Geometry: final body of the model. Coordinates: model frame, mm. A direction names the side the tool comes from. Give positions to 0.01 mm unless a question says otherwise; leave off trailing zeros. Write each loop counter-clockwise with the first axis right and the second up, starting at its lowest first coordinate (ties: lowest second). Pieces come first, ordered by that corner, then holes. Notation, with made-up numbers: (12, 22.5) -> (44, 22.5) arc R13 ccw to (44, 33.5) -> close; hole circle Ø8 at (43, 69.5). An arc over 180 degrees is marked (long way). Answer as a JSON object with one key per item and string values. Group by question number.
(1) Section query D-D on z = 1.75. Output: boundary loops of the cut face in (x, y).
(2) Set-up query: faces 4 (the face through (2, -2, 0)), 5 (the face through (-2, 2, 17)), 6 (the face through (-2.003, 0.631, 2.218)). Return all of +Z, -Z, +X, -X, +Y, -Y with unobstructed straight access to the full face (end or side cutting, diameter ignored); none if empty.
(3) Section query C-C on z = 7.5. Output: boundary loops of the cut face in (x, y), plus the area to 3 significant figures.
(4) Draft query along X for faces 1 (the face through (-3, 0, 20)), 2 (the face through (1, -1, 23)), 3 (the face through (0, -1, 14)). Return one class per face: +X half, -X half, draft (parallel to the pull), parting line (faces both ways), or undercut.
(5) Section query A-A on y = 0. Output: boundary loops of the cut face in (x, z), plus the area to 3 significant figures.
(6) Contact query for flat-ended pins moving along their axis: pin 1 Ø1.6 at (x, y) = (0, 0) entering from -Z; pin 2 Ø2 at (y, z) = (-0.5, 20.5) entering from -X; pin 3 Ø1.3 at (x, y) = (-0.5, 1) entering from -Z; pin 4 Ø1.5 at (x, z) = (1.5, 19) entering from +Y. Output: stop coordinate, or through.
(7) Material intervals for probe 1 along Y at (x, z) = (0, 12); probe 2 along Y at (x, z) = (0, 2.8); probe 3 along Z at (x, y) = (-1.5, 2.75), sorted ascending.
Autodesk Inventor part; units mm, degrees
ref_plane "YZ Plane" through (0, 0, 0) normal (1, 0, 0) x (0, 1, 0)
ref_plane "XZ Plane" through (0, 0, 0) normal (0, 1, 0) x (-1, 0, 0)
ref_plane "XY Plane" through (0, 0, 0) normal (0, 0, 1) x (1, 0, 0)
sketch "Sketch1" plane through (0, 0, 0) normal (0, 0, 1) x (1, 0, 0)
  circle A0 centre (0, 0) radius 3.5
  dimension "d0" = 7
extrude "Extrusion1" add sketch "Sketch1" along normal blind 15
sketch "Sketch2" plane through (0, 0, 15) normal (0, 0, 1) x (1, 0, 0)
  circle A0 centre (0, 0) radius 2.5
  dimension "d3" = 5
extrude "Extrusion2" add sketch "Sketch2" along normal blind 2
sketch "Sketch3" plane through (0, 0, 17) normal (0, 0, 1) x (1, 0, 0)
  circle A0 centre (0, 0) radius 3
  dimension "d6" = 6
extrude "Extrusion3" add sketch "Sketch3" along normal blind 6
sketch "Sketch4" plane through (0, 0, 23) normal (0, 0, 1) x (1, 0, 0)
  circle A0 centre (0, 0) radius 1
  dimension "d9" = 2
extrude "Extrusion4" cut sketch "Sketch4" against normal through all
thread "Thread1"
fillet "Fillet1" radius 0.5 1 edges at (-3, 0, 23)
sketch "Sketch5" plane through (0, 0, 0) normal (0, 0, -1) x (-1, 0, 0)
  circle A0 centre (0, 0) radius 2.1
  dimension "d15" = 4.2
extrude "Extrusion5" cut sketch "Sketch5" against normal blind 4.5
properties part number "nozzle throat" material "Stainless Steel"
Answer list:
{
 "1": {"outline": "circle Ø7 at (0, 0); hole circle Ø4.2 at (0, 0)"},
 "2": {"face 4": "-Z, +X, -X, +Y, -Y", "face 5": "none", "face 6": "-Z"},
 "3": {"outline": "circle Ø7 at (0, 0); hole circle Ø2 at (0, 0)", "area": "35.3 mm2"},
 "4": {"face 1": "parting line", "face 2": "draft", "face 3": "undercut"},
 "5": {"outline": "(-3.5, 0) -> (-2.1, 0) -> (-2.1, 4.5) -> (-1, 4.5) -> (-1, 23) -> (-2.5, 23) arc R0.5 ccw to (-3, 22.5) -> (-3, 17) -> (-2.5, 17) -> (-2.5, 15) -> (-3.5, 15) -> close; (1, 4.5) -> (2.1, 4.5) -> (2.1, 0) -> (3.5, 0) -> (3.5, 15) -> (2.5, 15) -> (2.5, 17) -> (3, 17) -> (3, 22.5) arc R0.5 ccw to (2.5, 23) -> (1, 23) -> close", "area": "95.0 mm2"},
 "6": {"pin 1": "through", "pin 2": "x = -3", "pin 3": "z = 4.5", "pin 4": "y = 2.9"},
 "7": {"probe 1": "-3.5 to -1, 1 to 3.5", "probe 2": "-3.5 to -2.1, 2.1 to 3.5", "probe 3": "0 to 15"}
}
